from build123d import *

# Parameters (mm, degrees)
F1_DEPTH = 38.1
F3_DEPTH = 106.172
F4_DEPTH = 85.598


with BuildPart() as f1:
    # F0 (on Front) → F1 (new body)
    with BuildSketch(Plane.XZ):
        Polygon((63.5, 42.791789), (0, 42.791789), (-63.5, 42.791789), (-63.5, -21.281976), (-0.006818, 0), (63.5, -19.196785), align=None)
    extrude(amount=F1_DEPTH)

    # F2 (on Right) → F3 (cut)
    with BuildSketch(Plane.YZ):
        Polygon((0, -20.257542), (0, 43.2841), (-38.183279, 43.2841), align=None)
    extrude(amount=-F3_DEPTH, mode=Mode.SUBTRACT)

    # F2 (on Right) → F4 (cut)
    with BuildSketch(Plane.YZ):
        Polygon((0, -20.257542), (0, 43.2841), (-38.183279, 43.2841), align=None)
    extrude(amount=F4_DEPTH, mode=Mode.SUBTRACT)


solid = f1.part
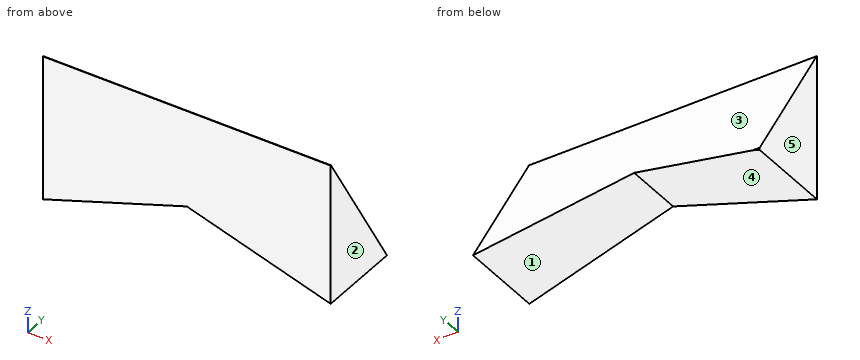
Read the model definition and answer for the solid it produces. Units are mm, in the model's axes. Face numbers are marked on the shaded views. A direction names the side the tool comes from. Round coordinates to 2 decimals unless told otherwise and drop trailing zeros. Write each loop counter-clockwise with the first axis right and the second up, starting at its lowest first coordinate (ties: lowest second). Pieces come first, ordered by that corner, then holes. Notation, with made-up numbers: (7, -6) - (28, -6) arc R19 cw to (28, 9) - close; hole circle Ø3 at (-30, -5.75). An arc over 180 degrees is marked (long way). One line per question, with ' | ' between items. Start each with the question number.
1. Section B-B (y = -10.5) is taken. Determine the outline of the cut face in (x, z).
2. Section D-D (x = -20) is taken. Determine the outline of the cut face in (y, z).
3. Find the intervals of material crossed by probe 1 along Y at (x, z) = (-39.5, 4.5); probe 2 along Z at (x, y) = (43, -33.5); probe 3 along Y at (x, z) = (-5, 23.5), in increasing order. Write a range as [from, to].
4. For a pull along X with two mould halves and no side action, classify the marked faces 1, 2 and 3 as +X half, -X half, draft (parallel to the pull), parting line (faces both ways), or undercut.
5. For the marked faces 4 and 5, determine the directions among +Z, -Z, +X, -X, +Y, -Y from which every point of the face is accessible in a straight line to the end or side of a thin tool.
6. Each of these flat-tipped pins is pushed along its axis until it touches: pin 1 (8 mm diameter, centred on x = -32, y = -25, fed in from -Z); pin 2 (8 mm diameter, centred on x = -22, y = -24.5, fed in from -Z). Where does it stop, or does it pass through?
7. Section C-C (y = -29) is taken. Determine the outline of the cut face in (x, z).
8. Section A-A (z = -7) is taken. Determine the outline of the cut face in (x, y).
Filled in:
1) outline: (-63.5, -21.28) - (-8.31, -2.78) - (-63.5, -2.78) - close; (9.2, -2.78) - (63.5, -19.2) - (63.5, -2.78) - close
2) outline: (-38.1, -6.7) - (-8.15, -6.7) - (-37.89, 42.79) - (-38.1, 42.79) - close
3) probe 1: [-38.1, -14.88] | probe 2: [-13, 35.49] | probe 3: [-38.1, -26.29]
4) face 1: undercut | face 2: +X half | face 3: draft
5) face 4: -Z, +Y, -Y | face 5: +Z, -Z, -X, +Y, -Y
6) pin 1: z = -12.06 | pin 2: z = -8.71
7) outline: (-63.5, -21.28) - (-0.01, 0) - (63.5, -19.2) - (63.5, 28) - (-63.5, 28) - close
8) outline: (-63.5, -38.1) - (-20.89, -38.1) - (-20.89, -7.97) - (-63.5, -7.97) - close; (23.15, -38.1) - (63.5, -38.1) - (63.5, -7.97) - (23.15, -7.97) - close
